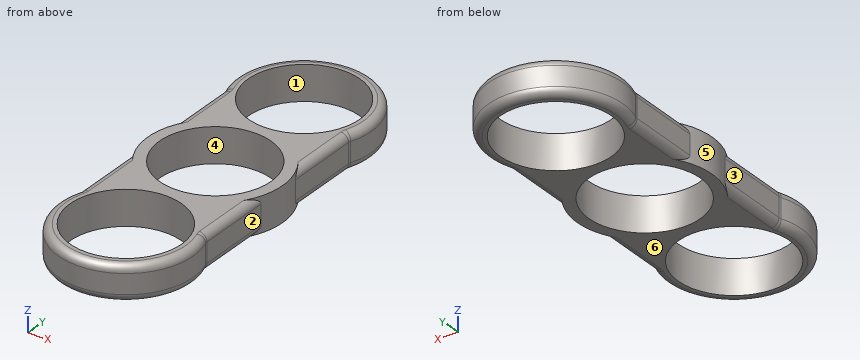
```python
from build123d import *

# Parameters (mm, degrees)
F0_R     = 11.2
F1_DEPTH = 7
F2_F1_R  = 1.5
F2_F2_R  = 1.5


with BuildPart() as f1:
    # F0 (on Top) → F1 (new body)
    with BuildSketch(Plane.XY):
        with BuildLine():
            Line((-12.5890504837, 19.9107848701), (-12.5890504837, 4.8750187608))
            ThreePointArc((-12.5890504837, 4.8750187608), (-13.4998898549, 0.0545335167), (-12.6280247824, -4.773153056))
            Line((-12.6280247824, -4.773153056), (-12.6280247824, -20.1613976912))
            ThreePointArc((-12.6280247824, -20.1613976912), (0, -38.4345507473), (12.6280247824, -20.1613976912))
            Line((12.6280247824, -20.1613976912), (12.6280247824, -4.773153056))
            ThreePointArc((12.6280247824, -4.773153056), (13.4998898549, 0.0545335167), (12.5890504837, 4.8750187608))
            Line((12.5890504837, 4.8750187608), (12.5890504837, 19.9107848701))
            ThreePointArc((12.5890504837, 19.9107848701), (0, 38.2858036309), (-12.5890504837, 19.9107848701))
        make_face()
        with Locations((0, -24.9345507473)):
            Circle(F0_R, mode=Mode.SUBTRACT)
        Circle(F0_R, mode=Mode.SUBTRACT)
        with Locations((0, 24.7858036309)):
            Circle(F0_R, mode=Mode.SUBTRACT)
    extrude(amount=F1_DEPTH)

    # F2: fillet of radius 1.5 on 8 edges, made by hand

    # F2_f1
    f2_f1_edges = [f1.edges().sort_by_distance(p)[0] for p in [
        (12.5890504837, 19.9107848701, 3.5),
        (-12.5890504837, 19.9107848701, 3.5),
        (-12.6280247824, -20.1613976912, 3.5),
        (12.6280247824, -20.1613976912, 3.5),
    ]]
    fillet(f2_f1_edges, radius=F2_F1_R)

    # F2_f2
    f2_f2_edges = [f1.edges().sort_by_distance(p)[0] for p in [
        (0, 38.2858036309, 0),
        (0, 38.2858036309, 7),
        (0, -38.4345507473, 0),
        (0, -38.4345507473, 7),
        (-12.6499849119, -20.1505476521, 7),
        (12.6499849119, -20.1505476521, 7),
        (-12.6499849119, -20.1505476521, 0),
        (12.6499849119, -20.1505476521, 0),
        (12.6119997783, 19.8995023273, 7),
        (-12.6119997783, 19.8995023273, 7),
        (12.6119997783, 19.8995023273, 0),
        (-12.6119997783, 19.8995023273, 0),
    ]]
    fillet(f2_f2_edges, radius=F2_F2_R)


solid = f1.part
```
Read the model definition and answer for the solid it produces. Units are mm, in the model's axes. Face numbers are marked on the shaded views. A direction names the side the tool comes from. Give positions to 0.01 mm unless a question says otherwise; leave off trailing zeros. Loops run counter-clockwise (first coordinate to the right, second up) from the corner with the lowest first, then second, coordinate; pieces in that order, holes last.
Item 1: Each of these flat-tipped pins is pushed along its axis until it touches: pin 1 Ø2 at (y, z) = (23, 5) entering from +X; pin 2 Ø1.2 at (y, z) = (15, 3) entering from +X; pin 3 Ø1.2 at (y, z) = (9.5, 4) entering from -X. Where does it stop, or does it pass through?
Item 2: For the marked faces 1, 2 and 3, determine the directions among +Z, -Z, +X, -X, +Y, -Y from which every point of the face is accessible in a straight line to the end or side of a thin tool.
Item 3: Find the intervals of material crossed by line 1 along Y through (x, z) = (-7.75, 5.5); line 2 along Y through (x, z) = (9.25, 2.75); line 3 along X through (y, z) = (-7, 4.25), in increasing order.
Item 4: The part is cut by section C-C (z = 0.75). Write down the section's boundary in (x, y), and give its area (3 significant figures).
Item 5: The part is cut by section D-D (y = -10.5). Write down the section's boundary in (x, z).
Item 6: The mould has two halves that part along X. Classify the marked faces 4, 5 and 6: released by +X, released by -X, zero draft, split by the parting line, or undercut.
Item 7: The part is cut by section A-A (y = 0). Write down the section's boundary in (x, z), and give its area (3 significant figures).
Item 8: The part is cut by section B-B (x = 0). Write down the section's boundary in (y, z), and give its area (3 significant figures).
Taken from the geometry:
1. pin 1: stops at x = 13.48
1. pin 2: stops at x = 12.59
1. pin 3: stops at x = -12.59
2. face 1: +Z, -Z
2. face 2: +Z, -Z, +X
2. face 3: +Z, -Z, -X
3. line 1: y = -35.99 to -33.02, -16.85 to -8.09, 8.09 to 16.7, 32.87 to 35.84
3. line 2: y = -34.77 to -31.25, -18.62 to -6.31, 6.31 to 18.47, 31.1 to 34.62
3. line 3: x = -12.63 to -8.74, 8.74 to 12.63
4. outline: (-12.53, -20.47) arc R13.3 ccw (long way) to (12.53, -20.47) arc R1.7 cw to (12.43, -19.89) - (12.43, -5.27) arc R13.5 ccw to (12.39, 5.37) - (12.39, 19.64) arc R1.7 cw to (12.49, 20.22) arc R13.3 ccw (long way) to (-12.49, 20.22) arc R1.7 cw to (-12.39, 19.64) - (-12.39, 5.37) arc R13.5 ccw to (-12.43, -5.27) - (-12.43, -19.89) arc R1.7 cw to start; hole circle Ø22.4 at (0, -24.93); hole circle Ø22.4 at (0, 0); hole circle Ø22.4 at (0, 24.79)
4. area: 634 mm2
5. outline: (-12.63, 1.5) arc R1.5 ccw to (-11.13, 0) - (-3.9, 0) - (-3.9, 7) - (-11.13, 7) arc R1.5 ccw to (-12.63, 5.5) - close; (3.9, 0) - (11.13, 0) arc R1.5 ccw to (12.63, 1.5) - (12.63, 5.5) arc R1.5 ccw to (11.13, 7) - (3.9, 7) - close
6. face 4: undercut
6. face 5: released by -X
6. face 6: zero draft
7. outline: (-13.5, 0) - (-11.2, 0) - (-11.2, 7) - (-13.5, 7) - close; (11.2, 0) - (13.5, 0) - (13.5, 7) - (11.2, 7) - close
7. area: 32.2 mm2
8. outline: (-38.43, 1.5) arc R1.5 ccw to (-36.93, 0) - (-36.13, 0) - (-36.13, 7) - (-36.93, 7) arc R1.5 ccw to (-38.43, 5.5) - close; (-13.73, 0) - (-11.2, 0) - (-11.2, 7) - (-13.73, 7) - close; (11.2, 0) - (13.59, 0) - (13.59, 7) - (11.2, 7) - close; (35.99, 0) - (36.79, 0) arc R1.5 ccw to (38.29, 1.5) - (38.29, 5.5) arc R1.5 ccw to (36.79, 7) - (35.99, 7) - close
8. area: 64.7 mm2
